Design review of the part built by this model. Coordinates are the model's own, in mm. A direction names the side the tool comes from. Coordinates: 2 decimals unless noted, no trailing zeros. Loops run counter-clockwise (first coordinate to the right, second up) from the corner with the lowest first, then second, coordinate; pieces in that order, holes last. Notation, with made-up numbers: (-34.5, 38.25) -> (-7.5, 38.25) arc R8 ccw to (-7.5, 51.25) -> close; hole circle Ø6 at (-6, 7.5). An arc over 180 degrees is marked (long way). Answer as a JSON object with one key per item and string values.
```python
from build123d import *

# Parameters (mm, degrees)
DODANIE_WYCI_GNI_CIE1_DEPTH      = 5
DODANIE_WYCI_GNI_CIE2_DEPTH      = 5
DODANIE_WYCI_GNI_CIE2_DEPTH_BACK = 90
SZKIC1_3_W                       = 10
SZKIC1_3_H                       = 10
WYTNIJ_WYCI_GNI_CIE1_DEPTH       = 323.646908993
WYTNIJ_WYCI_GNI_CIE2_DEPTH       = 4.5


with BuildPart() as part:
    # Szkic1 → Dodanie-wyci_gni_cie1 (new body)
    with BuildSketch(Plane(origin=(0, 0, 0), x_dir=(1, 0, 0), z_dir=(0, 1, 0))):
        with BuildLine():
            Line((10, 10), (10, 0))
            Line((10, 0), (270, 0))
            Line((270, 0), (270, 10))
            Line((270, 10), (280, 10))
            Line((280, 10), (280, 64.567847809))
            Line((280, 64.567847809), (116, 64.567847809))
            ThreePointArc((116, 64.567847809), (90, 38.567847809), (64, 64.567847809))
            Line((64, 64.567847809), (0, 64.567847809))
            Line((0, 64.567847809), (0, 10))
            Line((0, 10), (10, 10))
        make_face()
        with BuildLine():
            Line((0, 119.135695619), (0, 64.567847809))
            Line((0, 64.567847809), (64, 64.567847809))
            ThreePointArc((64, 64.567847809), (90, 90.567847809), (116, 64.567847809))
            Line((116, 64.567847809), (280, 64.567847809))
            Line((280, 64.567847809), (280, 119.135695619))
            Line((280, 119.135695619), (270, 119.135695619))
            Line((270, 119.135695619), (270, 129.135695619))
            Line((270, 129.135695619), (10, 129.135695619))
            Line((10, 129.135695619), (10, 119.135695619))
            Line((10, 119.135695619), (0, 119.135695619))
        make_face()
    extrude(amount=DODANIE_WYCI_GNI_CIE1_DEPTH)

    # Szkic1_3 → Dodanie-wyci_gni_cie2 (add, two sides: drawn at the far end of the back side and taken through both)
    with BuildSketch(Plane(origin=(0, 0, 0), x_dir=(1, 0, 0), z_dir=(0, 1, 0)).offset(-DODANIE_WYCI_GNI_CIE2_DEPTH_BACK)):
        with Locations((5, 5)):
            Rectangle(SZKIC1_3_W, SZKIC1_3_H)
        with Locations((275, 5)):
            Rectangle(SZKIC1_3_W, SZKIC1_3_H)
        with Locations((275, 124.135695619)):
            Rectangle(SZKIC1_3_W, SZKIC1_3_H)
        with Locations((5, 124.135695619)):
            Rectangle(SZKIC1_3_W, SZKIC1_3_H)
    extrude(amount=DODANIE_WYCI_GNI_CIE2_DEPTH + DODANIE_WYCI_GNI_CIE2_DEPTH_BACK)

    # Szkic2 → Wytnij-wyci_gni_cie1 (cut, through all)
    with BuildSketch(Plane(origin=(0, 5, 0), x_dir=(1, 0, 0), z_dir=(0, 1, 0))):
        with BuildLine():
            Line((174.634543985, 93.017847809), (234.634543985, 93.017847809))
            ThreePointArc((234.634543985, 93.017847809), (236.884543985, 95.267847809), (234.634543985, 97.517847809))
            Line((234.634543985, 97.517847809), (174.634543985, 97.517847809))
            ThreePointArc((174.634543985, 97.517847809), (172.384543985, 95.267847809), (174.634543985, 93.017847809))
        make_face()
        with BuildLine():
            ThreePointArc((234.634543985, 36.117847809), (236.884543985, 33.867847809), (234.634543985, 31.617847809))
            Line((234.634543985, 31.617847809), (174.634543985, 31.617847809))
            ThreePointArc((174.634543985, 31.617847809), (172.384543985, 33.867847809), (174.634543985, 36.117847809))
            Line((174.634543985, 36.117847809), (234.634543985, 36.117847809))
        make_face()
    extrude(amount=-WYTNIJ_WYCI_GNI_CIE1_DEPTH, mode=Mode.SUBTRACT)

    # Szkic2_3 → Wytnij-wyci_gni_cie2 (cut)
    # profile 1 of 2: a face of its own
    with BuildSketch(Plane(origin=(0, 5, 0), x_dir=(1, 0, 0), z_dir=(0, 1, 0))):
        with BuildLine():
            Line((174.634543985, 99.017847809), (234.634543985, 99.017847809))
            ThreePointArc((234.634543985, 99.017847809), (238.384543985, 95.267847809), (234.634543985, 91.517847809))
            Line((234.634543985, 91.517847809), (174.634543985, 91.517847809))
            ThreePointArc((174.634543985, 91.517847809), (170.884543985, 95.267847809), (174.634543985, 99.017847809))
        make_face()
        with BuildLine():
            Line((174.634543985, 97.517847809), (234.634543985, 97.517847809))
            ThreePointArc((234.634543985, 97.517847809), (236.884543985, 95.267847809), (234.634543985, 93.017847809))
            Line((234.634543985, 93.017847809), (174.634543985, 93.017847809))
            ThreePointArc((174.634543985, 93.017847809), (172.384543985, 95.267847809), (174.634543985, 97.517847809))
        make_face(mode=Mode.SUBTRACT)
    # profile 2 of 2: a face of its own
    with BuildSketch(Plane(origin=(0, 5, 0), x_dir=(1, 0, 0), z_dir=(0, 1, 0))):
        with BuildLine():
            Line((174.634543985, 30.117847809), (234.634543985, 30.117847809))
            ThreePointArc((234.634543985, 30.117847809), (238.384543985, 33.867847809), (234.634543985, 37.617847809))
            Line((234.634543985, 37.617847809), (174.634543985, 37.617847809))
            ThreePointArc((174.634543985, 37.617847809), (170.884543985, 33.867847809), (174.634543985, 30.117847809))
        make_face()
        with BuildLine():
            Line((174.634543985, 31.617847809), (234.634543985, 31.617847809))
            ThreePointArc((234.634543985, 31.617847809), (236.884543985, 33.867847809), (234.634543985, 36.117847809))
            Line((234.634543985, 36.117847809), (174.634543985, 36.117847809))
            ThreePointArc((174.634543985, 36.117847809), (172.384543985, 33.867847809), (174.634543985, 31.617847809))
        make_face(mode=Mode.SUBTRACT)
    extrude(amount=-WYTNIJ_WYCI_GNI_CIE2_DEPTH, mode=Mode.SUBTRACT)


solid = part.part
```
1) The part is to be moulded in two halves that separate along X. For faces 4 (the flat face through (0, 3, -64)), 5 (the flat face through (205.1, 0.5, -92.8)), 6 (the flat face through (138, 5, -65)), 7 (the flat face through (204.2, 0.5, -36.4)), say which applies: pulls with the +X half, pulls with the -X half, needs draft (parallel to the pull), parting line crosses it, or undercut.
Completed:
{"face 4": "pulls with the -X half", "face 5": "undercut", "face 6": "needs draft", "face 7": "undercut"}
2) Add section D-D, the plane z = -102. Give the boundary of the cut face in (x, y), and give its area (3 significant figures).
Completed:
{"outline": "(0, 0) -> (280, 0) -> (280, 5) -> (0, 5) -> close", "area": "1,400 mm²"}
3) For faces 1 (the flat face through (10, -46, -124)), 2 (the flat face through (275, -46, -10)), 3 (the flat face through (280, 3, -64)), list the 3-axis set-ups (+Z, -Z, +X, -X, +Y, -Y) from which the entire face can be reached by the end or side of a thin tool; tool diameter is ignored.
Completed:
{"face 1": "+Z, -Z, -Y", "face 2": "+X, -X, -Y", "face 3": "+Z, -Z, +X, +Y, -Y"}
4) Clearance check with a flat-ended pin moving along its axis: pin 1 Ø3 at (x, z) = (156.5, -73) entering from -Y. State where the tip first meets the part, or that it passes through.
Completed:
{"pin 1": "y = 0"}
5) Add section C-C, the plane x = 90. Give the boundary of the cut face in (y, z).
Completed:
{"outline": "(0, -129.14) -> (5, -129.14) -> (5, -90.57) -> (0, -90.57) -> close; (0, -38.57) -> (5, -38.57) -> (5, 0) -> (0, 0) -> close"}
6) Add section B-B, the plane x = 198.5. Give the boundary of the cut face in (y, z).
Completed:
{"outline": "(0, -129.14) -> (5, -129.14) -> (5, -99.02) -> (0.5, -99.02) -> (0.5, -97.52) -> (0, -97.52) -> close; (0, -93.02) -> (0.5, -93.02) -> (0.5, -91.52) -> (5, -91.52) -> (5, -37.62) -> (0.5, -37.62) -> (0.5, -36.12) -> (0, -36.12) -> close; (0, -31.62) -> (0.5, -31.62) -> (0.5, -30.12) -> (5, -30.12) -> (5, 0) -> (0, 0) -> close"}
7) Add section A-A, the plane y = -39. Give the boundary of the cut face in (x, z), and give its area (3 significant figures).
Completed:
{"outline": "(0, -129.14) -> (10, -129.14) -> (10, -119.14) -> (0, -119.14) -> close; (0, -10) -> (10, -10) -> (10, 0) -> (0, 0) -> close; (270, -129.14) -> (280, -129.14) -> (280, -119.14) -> (270, -119.14) -> close; (270, -10) -> (280, -10) -> (280, 0) -> (270, 0) -> close", "area": "400 mm²"}
8) Wall thickness on probe 1 along Z at (x, y) = (90, 2); probe 2 along Y at (x, z) = (141, -51.5): over which ranges is each line inside the solid? List them lowest first.
Completed:
{"probe 1": "-129.14 to -90.57, -38.57 to 0", "probe 2": "0 to 5"}
